Check sheet for the modelled part. Datum: model origin and axes. Units: mm. A direction names the side the tool comes from. Round coordinates to 2 decimals unless told otherwise and drop trailing zeros. Loops run counter-clockwise (first coordinate to the right, second up) from the corner with the lowest first, then second, coordinate; pieces in that order, holes last. Notation, with made-up numbers: (37, -39) -> (56, -39) arc R20 ccw to (56, -34) -> close; hole circle Ø8 at (77.25, 82). An arc over 180 degrees is marked (long way). One line per question, with ' | ' between items.
```python
from build123d import *

# Parameters (mm, degrees)
F0_R     = 5
F1_DEPTH = 17.5
F2_R     = 10
F3_DEPTH = 2
F4_R     = 2
F5_DEPTH = 25


# Not quite as in the source:
# - a pattern or mirror of a feature is missing from the dataset's text; its kind, count and spacing are read off the source's solid


with BuildPart() as f1:
    # F0 (on Front) → F1 (new body, symmetric)
    with BuildSketch(Plane.XZ):
        Polygon((20, 13), (0, 13), (-20, 13), (-20, 5), (-18, 3), (-18, -8), (-12, -8), (-7, -13), (0, -13), (7, -13), (12, -8), (18, -8), (18, 3), (20, 5), align=None)
        Circle(F0_R, mode=Mode.SUBTRACT)
    extrude(amount=F1_DEPTH, both=True)

    # F2 (on face) → F3 (cut)
    with BuildSketch(Plane.XZ.offset(17.5)):
        Circle(F2_R)
    f3 = extrude(amount=-F3_DEPTH, mode=Mode.SUBTRACT)

    # F3_copies: F3 across plane
    add(f3.mirror(Plane.ZX), mode=Mode.SUBTRACT)

    # F4 (on face) → F5 (cut)
    with BuildSketch(Plane.XY.offset(13)):
        with Locations((-14, 10.5)):
            Circle(F4_R)
        with Locations((-14, -10.5)):
            Circle(F4_R)
        with Locations((14, 10.5)):
            Circle(F4_R)
        with Locations((14, -10.5)):
            Circle(F4_R)
    extrude(amount=-F5_DEPTH, mode=Mode.SUBTRACT)


solid = f1.part
```
(1) Sectioned sample at B-B, the plane z = 0. Record the cut outline in (x, y).
Answer:
outline: (-18, -17.5) -> (-10, -17.5) -> (-10, -15.5) -> (-5, -15.5) -> (-5, 15.5) -> (-10, 15.5) -> (-10, 17.5) -> (-18, 17.5) -> close; (5, -15.5) -> (10, -15.5) -> (10, -17.5) -> (18, -17.5) -> (18, 17.5) -> (10, 17.5) -> (10, 15.5) -> (5, 15.5) -> close; hole circle Ø4 at (-14, -10.5); hole circle Ø4 at (-14, 10.5); hole circle Ø4 at (14, -10.5); hole circle Ø4 at (14, 10.5)
(2) Go/stop test with flat-tipped pins: pin 1 (6.5 mm diameter, centred on x = 15.5, y = -2.5, fed in from -Z); pin 2 (12 mm diameter, centred on y = -8, z = -5.5, fed in from +X); pin 3 (6 mm diameter, centred on x = 4, z = -2, fed in from +Y). Record where each tip stops, or that it passes through.
Answer:
pin 1: stops at z = -8 | pin 2: stops at x = 18 | pin 3: stops at y = 15.5
(3) Set-up check for faces 5 (the face through (-14.26, 12.483, 2.647)), 6 (the face through (15, 0, -8)), 7 (the face through (-5, 15.5, -2)): record each of +Z, -Z, +X, -X, +Y, -Y from which the full face is reachable in a straight line by a thin tool's end or side.
Answer:
face 5: +Z, -Z | face 6: -Z, +X, +Y, -Y | face 7: +Y
(4) Sectioned sample at A-A, the plane y = -11. Record the cut outline in (x, z), and give its area (3 significant figures).
Answer:
outline: (-20, 5) -> (-18, 3) -> (-18, -8) -> (-15.94, -8) -> (-15.94, 13) -> (-20, 13) -> close; (-12.06, -8) -> (-12, -8) -> (-7, -13) -> (7, -13) -> (12, -8) -> (12.06, -8) -> (12.06, 13) -> (-12.06, 13) -> close; (15.94, -8) -> (18, -8) -> (18, 3) -> (20, 5) -> (20, 13) -> (15.94, 13) -> close; hole circle Ø10 at (0, 0) | area: 646 mm2
(5) Mould release check, pull along X, two halves, no side actions. Record for faces 1 (the face through (-19, 0, 4)), 2 (the face through (-1.08, 0.22, -4.88)), 3 (the face through (-2.17, 16.51, -9.76)), 4 (the face through (18, 0, -3)): +X half, -X half, draft (parallel to the pull), parting line (faces both ways), or undercut.
Answer:
face 1: -X half | face 2: undercut | face 3: undercut | face 4: +X half
(6) Sectioned sample at C-C, the plane y = -7. Record the cut outline in (x, z).
Answer:
outline: (-20, 5) -> (-18, 3) -> (-18, -8) -> (-12, -8) -> (-7, -13) -> (7, -13) -> (12, -8) -> (18, -8) -> (18, 3) -> (20, 5) -> (20, 13) -> (-20, 13) -> close; hole circle Ø10 at (0, 0)
(7) Sectioned sample at D-D, the plane z = 10.75. Record the cut outline in (x, y).
Answer:
outline: (-20, -17.5) -> (20, -17.5) -> (20, 17.5) -> (-20, 17.5) -> close; hole circle Ø4 at (-14, -10.5); hole circle Ø4 at (-14, 10.5); hole circle Ø4 at (14, -10.5); hole circle Ø4 at (14, 10.5)
(8) Scan lines: probe 1 along X at (y, z) = (2, 0); probe 2 along X at (y, z) = (-9, -0.5); probe 3 along Y at (x, z) = (14, 8.25). Record each from-to range of solid material in increasing order.
Answer:
probe 1: x = -18 to -5, 5 to 18 | probe 2: x = -18 to -15.32, -12.68 to -4.97, 4.97 to 12.68, 15.32 to 18 | probe 3: y = -17.5 to -12.5, -8.5 to 8.5, 12.5 to 17.5
